Read the model definition and answer for the solid it produces. Units are mm, in the model's axes. A direction names the side the tool comes from. Give positions to 0.01 mm unless a question says otherwise; leave off trailing zeros. Loops run counter-clockwise (first coordinate to the right, second up) from the corner with the lowest first, then second, coordinate; pieces in that order, holes last. Notation, with made-up numbers: (57, -7.5) - (78, -7.5) arc R25 ccw to (78, 10.5) - close; hole circle Ø6 at (15, 81). An arc over 180 degrees is marked (long way). Write each question's results on one line, items separated by ' | '. Start each with the question number.
Q1. For faces 4 (the cylindrical face through (20.25, 1.48, -5.02)), 5 (the flat face through (30.5, -14, -10)), determine the directions among +Z, -Z, +X, -X, +Y, -Y from which every point of the face is accessible in a straight line to the end or side of a thin tool.
Q2. The part is cut by section C-C, the plane y = -17. Write down the section's boundary in (x, z), plus the area to 3 significant figures.
Q3. The part is cut by section A-A, the plane x = 15.25. Write down the section's boundary in (y, z).
Q4. Find the intervals of material crossed by line 1 (Z direction, x = 8, y = 1.65); line 2 (Y direction, x = 24.5, z = -15.75); line 3 (X direction, y = -27, z = -19.5), in increasing order. Write a range as from..to.
Q5. Given pin 1 (2 mm diameter, centred on x = 13, z = -5.5, fed in from -Y); pin 2 (5.5 mm diameter, centred on y = -17.5, z = -4.6, fed in from -X); pin 3 (2 mm diameter, centred on y = -17.5, z = -21.6, fed in from +X), each flat-ended and moving along its own axis, determine where each tip first touches the part or whether it passes through.
Q6. The part is cut by section D-D, the plane z = -4.6. Write down the section's boundary in (x, y).
Q7. Determine the mould class of faces 1 (the flat face through (21.6, 0.4, -26.2)), 2 (the cylindrical face through (17.557, 1.479, -17.536)), 3 (the flat face through (0, 1, -13)) for opening direction X: +X half, -X half, draft (parallel to the pull), parting line (faces both ways), or undercut.
Q8. The part is cut by section B-B, the plane x = 8. Write down the section's boundary in (y, z), plus the area to 3 significant figures.
```python
from build123d import *

# Parameters (mm, degrees)
SKETCH1_W               = 33.5
SKETCH1_H               = 26.2
BOSS_EXTRUDE1_DEPTH     = 3
SKETCH3_W               = 3
SKETCH3_H               = 26.2
BOSS_EXTRUDE3_DEPTH     = 30.5
FILLET1_R               = 13
SKETCH7_R               = 1.75
SKETCH7_R_2             = 5
CUT_EXTRUDE1_DEPTH      = 4
FILLET2_R               = 3
SKETCH10_R              = 1.75
SKETCH10_R_2            = 4
CUT_EXTRUDE2_DEPTH      = 1
CUT_EXTRUDE2_DEPTH_BACK = 3.5


with BuildPart() as part:
    # Sketch1 → Boss-Extrude1 (new body)
    with BuildSketch(Plane(origin=(0, 0, 0), x_dir=(1, 0, 0), z_dir=(0, 1, 0))):
        with Locations((16.75, 13.1)):
            Rectangle(SKETCH1_W, SKETCH1_H)
    extrude(amount=BOSS_EXTRUDE1_DEPTH)

    # Sketch3 → Boss-Extrude3 (add)
    with BuildSketch(Plane.XZ):
        with Locations((32, -13.1)):
            Rectangle(SKETCH3_W, SKETCH3_H)
    extrude(amount=BOSS_EXTRUDE3_DEPTH)

    # Fillet1
    fillet1_edges = [part.edges().sort_by_distance(p)[0] for p in [
        (32, -30.5, -26.2),
        (32, -30.5, 0),
    ]]
    fillet(fillet1_edges, radius=FILLET1_R)

    # Sketch7 → Cut-Extrude1 (cut, through all)
    with BuildSketch(Plane.XZ):
        with Locations((8, -5.211347336)):
            Circle(SKETCH7_R)
        with Locations((8, -21.211347336)):
            Circle(SKETCH7_R)
        with Locations((22, -21.1)):
            Circle(SKETCH7_R)
        with Locations((22, -5.1)):
            Circle(SKETCH7_R)
        with Locations((15.25, -13.1)):
            Circle(SKETCH7_R_2)
    extrude(amount=-CUT_EXTRUDE1_DEPTH, mode=Mode.SUBTRACT)

    # Fillet2
    fillet2_edges = [part.edges().sort_by_distance(p)[0] for p in [
        (33.5, 3, -13.1),
        (30.5, 0, -13.1),
    ]]
    fillet(fillet2_edges, radius=FILLET2_R)

    # Sketch10 → Cut-Extrude2 (cut, two sides)
    with BuildSketch(Plane(origin=(33.5, 0, 0), x_dir=(0, 0, -1), z_dir=(1, 0, 0))) as cut_extrude2_sk:
        with Locations((4.6, -17.5)):
            Circle(SKETCH10_R)
        with Locations((21.6, -17.5)):
            Circle(SKETCH10_R)
        with Locations((13.1, -17.5)):
            Circle(SKETCH10_R_2)
    extrude(amount=CUT_EXTRUDE2_DEPTH, mode=Mode.SUBTRACT)
    extrude(cut_extrude2_sk.sketch, amount=-CUT_EXTRUDE2_DEPTH_BACK, mode=Mode.SUBTRACT)


solid = part.part
```
Check sheet entries:
1) face 4: +Y, -Y | face 5: +Z, -Z, -X, -Y
2) outline: (30.5, -26.2) - (33.5, -26.2) - (33.5, -23.28) - (30.5, -23.28) - close; (30.5, -19.92) - (33.5, -19.92) - (33.5, -17.07) - (30.5, -17.07) - close; (30.5, -9.13) - (33.5, -9.13) - (33.5, -6.28) - (30.5, -6.28) - close; (30.5, -2.92) - (33.5, -2.92) - (33.5, 0) - (30.5, 0) - close | area: 34.7 mm^2
3) outline: (0, -26.2) - (3, -26.2) - (3, -18.1) - (0, -18.1) - close; (0, -8.1) - (3, -8.1) - (3, 0) - (0, 0) - close
4) line 1: z = -26.2..-22.96, -19.46..-6.96, -3.46..0 | line 2: y = 0..3 | line 3: x = 30.5..33.5
5) pin 1: stops at y = 0 | pin 2: stops at x = 30.5 | pin 3: passes through
6) outline: (0, 0) - (6.36, 0) - (6.36, 3) - (0, 3) - close; (9.64, 0) - (20.32, 0) - (20.32, 3) - (9.64, 3) - close; (23.68, 0) - (27.5, 0) arc R3 cw to (30.5, -3) - (30.5, -15.75) - (33.5, -15.75) - (33.5, 0) arc R3 ccw to (30.5, 3) - (23.68, 3) - close; (30.5, -27.42) - (33.5, -27.42) - (33.5, -19.25) - (30.5, -19.25) - close
7) face 1: draft | face 2: undercut | face 3: -X half
8) outline: (0, -26.2) - (3, -26.2) - (3, -22.96) - (0, -22.96) - close; (0, -19.46) - (3, -19.46) - (3, -6.96) - (0, -6.96) - close; (0, -3.46) - (3, -3.46) - (3, 0) - (0, 0) - close | area: 57.6 mm^2
